Verification items for the finished model (mm, model axes). A direction names the side the tool comes from. Give positions to 0.01 mm unless a question says otherwise; leave off trailing zeros. Loops run counter-clockwise (first coordinate to the right, second up) from the corner with the lowest first, then second, coordinate; pieces in that order, holes last. Notation, with made-up numbers: M 89.5,-38.75 L 128.5,-38.75 A33 cw 128.5,-4.75 Z; hole C -8.75,-30.75 d2. An arc over 180 degrees is marked long. Use a Markdown table: item, result.
from build123d import *

# Parameters (mm, degrees)
BOSS_EXTRUDE1_DEPTH = 4
CUT_EXTRUDE1_START  = -1.7
CUT_EXTRUDE1_DEPTH  = 18.388140952
CUT_EXTRUDE2_DEPTH  = 20.088140952
SKETCH11_R          = 2.1
CUT_EXTRUDE4_DEPTH  = 20.088140952
CHAMFER1_SIZE       = 1.25
CUT_EXTRUDE5_DEPTH  = 5.5
SKETCH13_R          = 2.1
BOSS_EXTRUDE4_DEPTH = 0.5
CHAMFER3_SIZE       = 0.5


with BuildPart() as part:
    # Sketch1 → Boss-Extrude1 (new body)
    with BuildSketch(Plane(origin=(0, 1.7, 0), x_dir=(1, 0, 0), z_dir=(0, 1, 0))):
        with BuildLine():
            Line((-13.265, 4.98), (-13.265, -7.46))
            ThreePointArc((-13.265, -7.46), (-11.604295449, -11.469295449), (-7.595, -13.13))
            Line((-7.595, -13.13), (7.595, -13.13))
            ThreePointArc((7.595, -13.13), (11.604295449, -11.469295449), (13.265, -7.46))
            Line((13.265, -7.46), (13.265, 4.98))
            ThreePointArc((13.265, 4.98), (11.604295449, 8.989295449), (7.595, 10.65))
            Line((7.595, 10.65), (-7.595, 10.65))
            ThreePointArc((-7.595, 10.65), (-11.604295449, 8.989295449), (-13.265, 4.98))
        make_face()
    extrude(amount=-BOSS_EXTRUDE1_DEPTH)

    # Sketch5 → Cut-Extrude1 (cut, through all)
    with BuildSketch(Plane(origin=(0, 1.7, 0), x_dir=(1, 0, 0), z_dir=(0, 1, 0)).offset(CUT_EXTRUDE1_START)):
        with BuildLine():
            Line((-7.595, -10.48), (7.595, -10.48))
            ThreePointArc((7.595, -10.48), (9.730462479, -9.595462479), (10.615, -7.46))
            Line((10.615, -7.46), (10.615, 4.98))
            ThreePointArc((10.615, 4.98), (9.730462479, 7.115462479), (7.595, 8))
            Line((7.595, 8), (-7.595, 8))
            ThreePointArc((-7.595, 8), (-9.730462479, 7.115462479), (-10.615, 4.98))
            Line((-10.615, 4.98), (-10.615, -7.46))
            ThreePointArc((-10.615, -7.46), (-9.730462479, -9.595462479), (-7.595, -10.48))
        make_face()
    extrude(amount=-CUT_EXTRUDE1_DEPTH, mode=Mode.SUBTRACT)

    # Sketch7 → Cut-Extrude2 (cut, through all)
    with BuildSketch(Plane(origin=(0, 1.7, 0), x_dir=(1, 0, 0), z_dir=(0, 1, 0))):
        with BuildLine():
            Line((2.2, -2.2), (2.2, 2.2))
            ThreePointArc((2.2, 2.2), (1.907106781, 2.907106781), (1.2, 3.2))
            Line((1.2, 3.2), (-1.2, 3.2))
            ThreePointArc((-1.2, 3.2), (-1.907106781, 2.907106781), (-2.2, 2.2))
            Line((-2.2, 2.2), (-2.2, -2.2))
            ThreePointArc((-2.2, -2.2), (-1.907106781, -2.907106781), (-1.2, -3.2))
            Line((-1.2, -3.2), (1.2, -3.2))
            ThreePointArc((1.2, -3.2), (1.907106781, -2.907106781), (2.2, -2.2))
        make_face()
    extrude(amount=-CUT_EXTRUDE2_DEPTH, mode=Mode.SUBTRACT)

    # Sketch11 → Cut-Extrude4 (cut, through all)
    with BuildSketch(Plane(origin=(0, 1.7, 0), x_dir=(1, 0, 0), z_dir=(0, 1, 0))):
        with Locations(Location((-7.615, 5.15, 0), (0, 0, 270))):
            Circle(SKETCH11_R)
        with Locations(Location((7.615, 5.15, 0), (0, 0, 270))):
            Circle(SKETCH11_R)
    extrude(amount=-CUT_EXTRUDE4_DEPTH, mode=Mode.SUBTRACT)

    # Chamfer1
    # the kernel refuses this chamfer: 1.25 mm, written as the material it adds along each edge
    with BuildSketch(Plane(origin=(-7.595, 0, 7.46), x_dir=(-1, 0, 0), z_dir=(0, 0, -1))) as chamfer1_piece_1:
        Polygon((3.02, -CHAMFER1_SIZE), (3.02 - CHAMFER1_SIZE, 0), (3.02, 0), align=None)
    revolve(axis=Axis((-7.595, 0, 7.46), (0, 1, 0)), revolution_arc=90)
    with BuildSketch(Plane(origin=(-7.595, 0, 10.48), x_dir=(0, -0.9996219169112968, 0.027495876610586317), z_dir=(1, 0, 0))) as chamfer1_piece_2:
        Polygon((CHAMFER1_SIZE * 0.999621916911, CHAMFER1_SIZE * 0.0274958766106), (-CHAMFER1_SIZE * 0.0274958766106, CHAMFER1_SIZE * 0.999621916911), (0, 0), align=None)
    extrude(amount=15.19)
    with BuildSketch(Plane(origin=(7.595, 0, 7.46), x_dir=(0, 0, 1), z_dir=(-1, 0, 0))) as chamfer1_piece_3:
        Polygon((3.02, -CHAMFER1_SIZE), (3.02 - CHAMFER1_SIZE, 0), (3.02, 0), align=None)
    revolve(axis=Axis((7.595, 0, 7.46), (0, 1, 0)), revolution_arc=90)
    with BuildSketch(Plane(origin=(10.615, 0, 7.46), x_dir=(0.027495876610586317, -0.9996219169112968, 0), z_dir=(0, 0, -1))) as chamfer1_piece_4_section:
        Polygon((CHAMFER1_SIZE * 0.999621916911, CHAMFER1_SIZE * 0.0274958766106), (-CHAMFER1_SIZE * 0.0274958766106, CHAMFER1_SIZE * 0.999621916911), (0, 0), align=None)
    chamfer1_piece_4 = extrude(amount=12.44, mode=Mode.PRIVATE)
    chamfer1_piece_4 = chamfer1_piece_4 - Plane(origin=(7.615, -0.413583305, -5.15), x_dir=(0, 0, 1), z_dir=(0, 1, 0)) * Cylinder(2.1, 30, mode=Mode.PRIVATE)
    add(chamfer1_piece_4)
    with BuildSketch(Plane(origin=(7.595, 0, -4.98), x_dir=(1, 0, 0), z_dir=(0, 0, 1))) as chamfer1_piece_5_section:
        Polygon((3.02, -CHAMFER1_SIZE), (3.02 - CHAMFER1_SIZE, 0), (3.02, 0), align=None)
    chamfer1_piece_5 = revolve(axis=Axis((7.595, 0, -4.98), (0, 1, 0)), revolution_arc=90, mode=Mode.PRIVATE)
    chamfer1_piece_5 = chamfer1_piece_5 - Plane(origin=(7.615, -0.471032406, -5.15), x_dir=(0, 0, 1), z_dir=(0, 1, 0)) * Cylinder(2.1, 13, mode=Mode.PRIVATE)
    add(chamfer1_piece_5)
    with BuildSketch(Plane(origin=(7.595, 0, -8), x_dir=(0, -0.9996219169112968, -0.027495876610586317), z_dir=(-1, 0, 0))) as chamfer1_piece_6_section:
        Polygon((CHAMFER1_SIZE * 0.999621916911, CHAMFER1_SIZE * 0.0274958766106), (-CHAMFER1_SIZE * 0.0274958766106, CHAMFER1_SIZE * 0.999621916911), (0, 0), align=None)
    chamfer1_piece_6 = extrude(amount=15.19, mode=Mode.PRIVATE)
    chamfer1_piece_6 = chamfer1_piece_6 - Plane(origin=(-7.615, -0.417580446, -5.15), x_dir=(0, 0, 1), z_dir=(0, 1, 0)) * Cylinder(2.1, 36, mode=Mode.PRIVATE)
    chamfer1_piece_6 = chamfer1_piece_6 - Plane(origin=(7.615, -0.417580446, -5.15), x_dir=(0, 0, 1), z_dir=(0, 1, 0)) * Cylinder(2.1, 36, mode=Mode.PRIVATE)
    add(chamfer1_piece_6)
    with BuildSketch(Plane(origin=(-7.595, 0, -4.98), x_dir=(0, 0, -1), z_dir=(1, 0, 0))) as chamfer1_piece_7_section:
        Polygon((3.02, -CHAMFER1_SIZE), (3.02 - CHAMFER1_SIZE, 0), (3.02, 0), align=None)
    chamfer1_piece_7 = revolve(axis=Axis((-7.595, 0, -4.98), (0, 1, 0)), revolution_arc=90, mode=Mode.PRIVATE)
    chamfer1_piece_7 = chamfer1_piece_7 - Plane(origin=(-7.615, -0.471032404, -5.15), x_dir=(0, 0, 1), z_dir=(0, 1, 0)) * Cylinder(2.1, 13, mode=Mode.PRIVATE)
    add(chamfer1_piece_7)
    with BuildSketch(Plane(origin=(-10.615, 0, -4.98), x_dir=(-0.027495876610586317, -0.9996219169112968, 0), z_dir=(0, 0, 1))) as chamfer1_piece_8_section:
        Polygon((CHAMFER1_SIZE * 0.999621916911, CHAMFER1_SIZE * 0.0274958766106), (-CHAMFER1_SIZE * 0.0274958766106, CHAMFER1_SIZE * 0.999621916911), (0, 0), align=None)
    chamfer1_piece_8 = extrude(amount=12.44, mode=Mode.PRIVATE)
    chamfer1_piece_8 = chamfer1_piece_8 - Plane(origin=(-7.615, -0.413583304, -5.15), x_dir=(0, 0, 1), z_dir=(0, 1, 0)) * Cylinder(2.1, 30, mode=Mode.PRIVATE)
    add(chamfer1_piece_8)

    # Sketch12 → Cut-Extrude5 (cut, symmetric)
    with BuildSketch(Plane.XY.offset(1.24)):
        Polygon((11.79, -2.45), (13.415, -2.45), (13.415, 1.85), (10.94, 1.85), (10.94, 0.45), (11.79, 0.45), (11.79, -1.125), (10.615, -2.3), (11.79, -2.3), align=None)
    cut_extrude5 = extrude(amount=CUT_EXTRUDE5_DEPTH, both=True, mode=Mode.SUBTRACT)

    # Mirror1: Cut-Extrude5 across plane
    add(cut_extrude5.mirror(Plane(origin=(0, 0, 0), x_dir=(0, 0, 1), z_dir=(1, 0, 0))), mode=Mode.SUBTRACT)

    # Sketch13 → Boss-Extrude4 (add)
    with BuildSketch(Plane(origin=(0, 1.7, 0), x_dir=(1, 0, 0), z_dir=(0, 1, 0))):
        with Locations(Location((7.615, 5.15, 0), (0, 0, 270))):
            Circle(SKETCH13_R)
        with Locations(Location((-7.615, 5.15, 0), (0, 0, 270))):
            Circle(SKETCH13_R)
    extrude(amount=-BOSS_EXTRUDE4_DEPTH)

    # Chamfer3
    chamfer3_edges = [part.edges().sort_by_distance(p)[0] for p in [
        (-13.265, 1.7, -4.62),
        (-11.604295449, 1.7, -8.989295449),
        (13.265, 1.7, -4.62),
        (10.94, 1.7, 1.24),
        (12.1025, 1.7, 6.74),
        (12.1025, 1.7, -4.26),
        (-13.265, 1.7, 7.1),
        (-10.94, 1.7, 1.24),
        (-12.1025, 1.7, 6.74),
        (-12.1025, 1.7, -4.26),
        (-1.907106781, 1.7, 2.907106781),
        (0, 1.7, 3.2),
        (1.907106781, 1.7, 2.907106781),
        (2.2, 1.7, 0),
        (1.907106781, 1.7, -2.907106781),
        (0, 1.7, -3.2),
        (0, 1.7, -10.65),
        (-1.907106781, 1.7, -2.907106781),
        (-2.2, 1.7, 0),
        (11.604295449, 1.7, -8.989295449),
        (13.265, 1.7, 7.1),
        (11.604295449, 1.7, 11.469295449),
        (0, 1.7, 13.13),
        (-11.604295449, 1.7, 11.469295449),
    ]]
    chamfer(chamfer3_edges, length=CHAMFER3_SIZE)


solid = part.part
(1) Material ranges on line 1 (X direction, y = 0.8, z = -5.15) (3 decimals); line 2 (X direction, y = 0.7, z = -2.25); line 3 (Z direction, x = 4.5, y = -1.75), recorded low to high.
Results below:
| item | result |
|---|---|
| line 1 | -13.262 to -9.715, -5.515 to 5.515, 9.715 to 13.262 |
| line 2 | -10.94 to -2.2, 2.2 to 10.94 |
| line 3 | -10.65 to -8, 10.48 to 13.13 |
(2) Cross-section at A-A on z = 1.5. Record the cut outline in (x, y) (3 decimals), then the cut area to 3 significant figures.
Results below:
| item | result |
|---|---|
| outline | M -11.79,-1.125 L -10.615,-2.3 L -10.615,-1.25 L -9.365,0 L -2.2,0 L -2.2,1.2 L -2.7,1.7 L -10.44,1.7 L -10.94,1.2 L -10.94,0.45 L -11.79,0.45 Z; M 2.2,0 L 9.365,0 L 10.615,-1.25 L 10.615,-2.3 L 11.79,-1.125 L 11.79,0.45 L 10.94,0.45 L 10.94,1.2 L 10.44,1.7 L 2.7,1.7 L 2.2,1.2 Z |
| area | 35.6 mm^2 |
(3) Set-up check for faces 5 (the flat face through (0, 1, 3.2)), 6 (the cylindrical face through (9.707, -1.768, 9.619)), 7 (the flat face through (11.211, -1.704, 1.317)), 8 (the flat face through (-11.4, 0.45, 1.3)): record each of +Z, -Z, +X, -X, +Y, -Y from which the full face is reachable in a straight line by a thin tool's end or side.
Results below:
| item | result |
|---|---|
| face 5 | +Y, -Y |
| face 6 | -Y |
| face 7 | +X, -Y |
| face 8 | -X, +Y |
(4) Draft check along X on faces 1 (the flat face through (-2.2, 1, 0)), 2 (the cylindrical face through (-11.56, -0.526, -9.033)), 3 (the cylindrical face through (-8.89, 0.55, -6.82)), 4 (the cylindrical face through (11.648, -0.526, -8.945)). Enter one of: +X half, -X half, draft (parallel to the pull), parting line (faces both ways), or undercut.
Results below:
| item | result |
|---|---|
| face 1 | undercut |
| face 2 | -X half |
| face 3 | undercut |
| face 4 | +X half |
(5) Gauge pin test, flat ends, axial feed: P1, Ø5, axis at x = 7.615, z = -5.15, coming from the -Y side; P2, Ø5, axis at x = 9.5, z = -1, coming from the -Y side; P3, Ø3.5, axis at x = -7.615, z = -5.15, coming from the -Y side. Record the tip position at first contact, or that the pin passes through.
Results below:
| item | result |
|---|---|
| P1 | y = -0.9 |
| P2 | y = -2.3 |
| P3 | y = 1.2 |
(6) Cross-section at D-D on x = 7. Record the cut outline in (y, z).
Results below:
| item | result |
|---|---|
| outline | M -2.3,-10.65 L 1.2,-10.65 L 1.7,-10.15 L 1.7,12.63 L 1.2,13.13 L -2.3,13.13 L -2.3,10.48 L -1.25,10.48 L 0,9.23 L 0,-3.14 L 1.2,-3.14 L 1.2,-7.16 L -0.41,-7.16 L -1.25,-8 L -2.3,-8 Z |
(7) Cross-section at B-B on x = -4. Record the cut outline in (y, z), then the cut area to 3 significant figures.
Results below:
| item | result |
|---|---|
| outline | M -2.3,-10.65 L 1.2,-10.65 L 1.7,-10.15 L 1.7,12.63 L 1.2,13.13 L -2.3,13.13 L -2.3,10.48 L -1.25,10.48 L 0,9.23 L 0,-6.75 L -1.25,-8 L -2.3,-8 Z |
| area | 53.9 mm^2 |
(8) Cross-section at C-C on z = 5.25. Record the cut outline in (x, y) (3 decimals).
Results below:
| item | result |
|---|---|
| outline | M -11.79,-1.125 L -10.615,-2.3 L -10.615,-1.25 L -9.365,0 L 9.365,0 L 10.615,-1.25 L 10.615,-2.3 L 11.79,-1.125 L 11.79,0.45 L 10.94,0.45 L 10.94,1.2 L 10.44,1.7 L -10.44,1.7 L -10.94,1.2 L -10.94,0.45 L -11.79,0.45 Z |
